Can you work these out from the model? Positions are in its coordinate system, mm. Give positions to 0.01 mm unless a question says otherwise; leave off trailing zeros. Loops run counter-clockwise (first coordinate to the right, second up) from the corner with the lowest first, then second, coordinate; pieces in that order, holes last. Notation, with made-up numbers: (74.5, 79.25) -> (98.5, 79.25) arc R20 cw to (98.5, 84.25) -> close; hole circle Ø3 at (0.5, 76.25). An arc over 180 degrees is marked (long way). One line per question, with ' | ' between items.
from build123d import *

# Parameters (mm, degrees)
SKETCH1_W           = 3
SKETCH1_H           = 15
SKETCH1_W_2         = 112
SKETCH1_H_2         = 40
SKETCH1_W_3         = 20
SKETCH1_H_3         = 3
BOSS_EXTRUDE1_DEPTH = 3
SKETCH2_W           = 112
SKETCH2_H           = 4
CUT_EXTRUDE1_DEPTH  = 3


with BuildPart() as part:
    # Sketch1 → Boss-Extrude1 (new body)
    with BuildSketch(Plane.XY):
        with Locations((-57.5, 0)):
            Rectangle(SKETCH1_W, SKETCH1_H)
        Rectangle(SKETCH1_W_2, SKETCH1_H_2)
        with Locations((-35, -21.5)):
            Rectangle(SKETCH1_W_3, SKETCH1_H_3)
        with Locations((0, -21.5)):
            Rectangle(SKETCH1_W_3, SKETCH1_H_3)
        with Locations((35, -21.5)):
            Rectangle(SKETCH1_W_3, SKETCH1_H_3)
        with Locations((57.5, 0)):
            Rectangle(SKETCH1_W, SKETCH1_H)
    extrude(amount=BOSS_EXTRUDE1_DEPTH)

    # Sketch2 → Cut-Extrude1 (cut)
    with BuildSketch(Plane.XY.offset(3)):
        with Locations((0, 18)):
            Rectangle(SKETCH2_W, SKETCH2_H)
    extrude(amount=-CUT_EXTRUDE1_DEPTH, mode=Mode.SUBTRACT)


solid = part.part
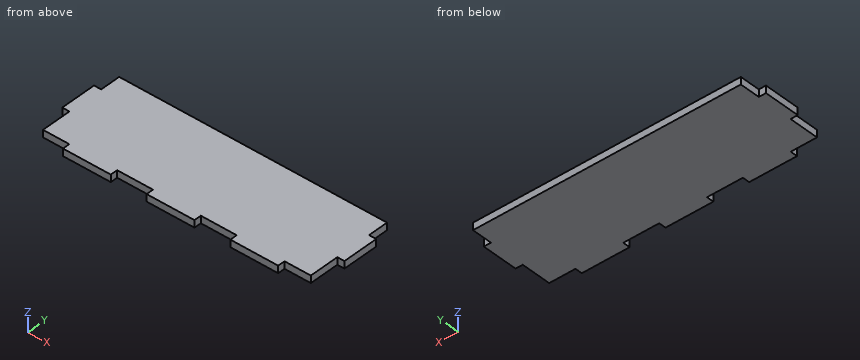
Q1. For pin 1 Ø1.5 at (y, z) = (11.5, 1) entering from +X; pin 2 Ø1.5 at (x, z) = (-50.5, 1.5) entering from -Y; pin 3 Ø0.9 at (y, z) = (-16.5, 1.5) entering from -X, each with a flat end and sliding along its axis, tell me the tip position at first contact or that it passes through.
Entries:
pin 1: x = 56 | pin 2: y = -20 | pin 3: x = -56
Q2. If we section it at B-B (y = -10): Write out the boundary of the cut face in (x, z), plus the area to 3 significant figures.
Entries:
outline: (-56, 0) -> (56, 0) -> (56, 3) -> (-56, 3) -> close | area: 336 mm²
Q3. If we section it at A-A (z = 1.9): Write out the boundary of the cut face in (x, y), plus the area to 3 significant figures.
Entries:
outline: (-59, -7.5) -> (-56, -7.5) -> (-56, -20) -> (-45, -20) -> (-45, -23) -> (-25, -23) -> (-25, -20) -> (-10, -20) -> (-10, -23) -> (10, -23) -> (10, -20) -> (25, -20) -> (25, -23) -> (45, -23) -> (45, -20) -> (56, -20) -> (56, -7.5) -> (59, -7.5) -> (59, 7.5) -> (56, 7.5) -> (56, 16) -> (-56, 16) -> (-56, 7.5) -> (-59, 7.5) -> close | area: 4,300 mm²
Q4. If I drill on probe 1 along X at (y, z) = (10, 0.75); probe 2 along Y at (x, z) = (-51.5, 1.1), over which ranges is the centre line in solid material (lowest first)? Write a range as from..to.
Entries:
probe 1: -56..56 | probe 2: -20..16
Q5. If we section it at C-C (x = 24): Write out the boundary of the cut face in (y, z), plus the area to 3 significant figures.
Entries:
outline: (-20, 0) -> (16, 0) -> (16, 3) -> (-20, 3) -> close | area: 108 mm²
